For this review, take the finished solid that the model builds, in its own axes (mm). A direction names the side the tool comes from. Round coordinates to 2 decimals unless told otherwise and drop trailing zeros. Order: outer loops, then holes, each group sorted by start corner. A loop starts at its lowest first (then second) coordinate and runs counter-clockwise, first axis right, second up. Notation, with made-up numbers: M -12,75 L 26,75 A24 cw 26,114 Z; hole C 1,19 d7. An arc over 180 degrees is marked long. Answer in a Markdown table with one row per item. Add a question column.
```python
from build123d import *

# Parameters (mm, degrees)
ESQUISSE1_R                         = 20
BOSS_EXTRU_1_DEPTH                  = 430.4
TROU_TARAUD_M81_D                   = 6.8
TROU_TARAUD_M81_DEPTH               = 22.25
TROU_TARAUD_M81_TIP                 = 2.042926105
ENL_V_MAT_EXTRU_1_REACH             = 433.328
ENL_V_MAT_EXTRU_1_DIRECTION_2_DEPTH = 432.328366793
TROU_TARAUD_M41_D                   = 3.3
TROU_TARAUD_M41_DEPTH               = 11.5
TROU_TARAUD_M41_TIP                 = 0.991420021
CHANFREIN1_SIZE                     = 0.8


with BuildPart() as part:
    # Esquisse1 → Boss.-Extru.1 (new body)
    with BuildSketch(Plane(origin=(0, 0, 0), x_dir=(1, 0, 0), z_dir=(0, 1, 0))):
        with Locations(Location((0, 0, 0), (0, 0, 90))):
            Circle(ESQUISSE1_R)
    extrude(amount=BOSS_EXTRU_1_DEPTH)

    # Trou taraudé M81
    with Locations(Plane(origin=(0, 0, 0), x_dir=(-1, 0, 0), z_dir=(0, -1, 0))):
        with Locations((0, -12.5), (0, 12.5)):
            Hole(TROU_TARAUD_M81_D / 2, depth=TROU_TARAUD_M81_DEPTH)
            with Locations((0, 0, -(TROU_TARAUD_M81_DEPTH + TROU_TARAUD_M81_TIP / 2))):  # 118° drill point
                Cone(0, TROU_TARAUD_M81_D / 2, TROU_TARAUD_M81_TIP, mode=Mode.SUBTRACT)

    # Esquisse8 → Enlèv. mat.-Extru.1 (cut, up to next)
    with BuildSketch(Plane.XZ, mode=Mode.PRIVATE) as enl_v_mat_extru_1_sk1:
        with BuildLine():
            Line((-5.5, 19.228884523), (-5.5, 18.9))
            Line((-5.5, 18.9), (5.5, 18.9))
            Line((5.5, 18.9), (5.5, 19.228884523))
            ThreePointArc((5.5, 19.228884523), (0, 20), (-5.5, 19.228884523))
        make_face()
    enl_v_mat_extru_1_tool1 = extrude(enl_v_mat_extru_1_sk1.sketch, amount=-ENL_V_MAT_EXTRU_1_REACH, mode=Mode.PRIVATE) & part.part
    # Esquisse8 → Enlèv. mat.-Extru.1 (cut, up to next)
    with BuildSketch(Plane.XZ, mode=Mode.PRIVATE) as enl_v_mat_extru_1_sk2:
        with BuildLine():
            Line((19.078784028, 6), (15, 6))
            Line((15, 6), (15, -6))
            Line((15, -6), (19.078784028, -6))
            ThreePointArc((19.078784028, -6), (20, 0), (19.078784028, 6))
        make_face()
    enl_v_mat_extru_1_tool2 = extrude(enl_v_mat_extru_1_sk2.sketch, amount=-ENL_V_MAT_EXTRU_1_REACH, mode=Mode.PRIVATE) & part.part
    add(enl_v_mat_extru_1_tool1.solids().sort_by_distance((0, 0, 19.353586))[0], mode=Mode.SUBTRACT)
    add(enl_v_mat_extru_1_tool2.solids().sort_by_distance((17.355884, 0, 0))[0], mode=Mode.SUBTRACT)

    # Esquisse8 → Enlèv. mat.-Extru.1 direction 2 (cut)
    with BuildSketch(Plane.XZ):
        with BuildLine():
            Line((-5.5, 19.228884523), (-5.5, 18.9))
            Line((-5.5, 18.9), (5.5, 18.9))
            Line((5.5, 18.9), (5.5, 19.228884523))
            ThreePointArc((5.5, 19.228884523), (0, 20), (-5.5, 19.228884523))
        make_face()
        with BuildLine():
            Line((19.078784028, 6), (15, 6))
            Line((15, 6), (15, -6))
            Line((15, -6), (19.078784028, -6))
            ThreePointArc((19.078784028, -6), (20, 0), (19.078784028, 6))
        make_face()
    extrude(amount=ENL_V_MAT_EXTRU_1_DIRECTION_2_DEPTH, mode=Mode.SUBTRACT)

    # Trou taraudé M41
    with Locations(Plane(origin=(15, 0, 0), x_dir=(0, 0, -1), z_dir=(1, 0, 0))):
        with Locations((0, 426.4)):
            Hole(TROU_TARAUD_M41_D / 2, depth=TROU_TARAUD_M41_DEPTH)
            with Locations((0, 0, -(TROU_TARAUD_M41_DEPTH + TROU_TARAUD_M41_TIP / 2))):  # 118° drill point
                Cone(0, TROU_TARAUD_M41_D / 2, TROU_TARAUD_M41_TIP, mode=Mode.SUBTRACT)

    # Chanfrein1
    chanfrein1_edges = [part.edges().sort_by_distance(p)[0] for p in [
        (5.5, 430.4, 19.064442262),
        (0, 430.4, 18.9),
        (-5.5, 430.4, 19.064442262),
        (-14.325501649, 430.4, -13.956360647),
        (17.039392014, 430.4, -6),
        (15, 430.4, 0),
        (17.039392014, 430.4, 6),
        (13.956360647, 430.4, 14.325501649),
    ]]
    chamfer(chanfrein1_edges, length=CHANFREIN1_SIZE)


solid = part.part
```
1. The part is to be moulded in two halves that separate along Z. For faces 4 (the conical face through (13.583, 430.272, 13.75)), 5 (the flat face through (-1, 0, 0)), 6 (the cylindrical face through (-0.74, 11.28, 15.82)), say which applies: pulls with the +Z half, pulls with the -Z half, needs draft (parallel to the pull), parting line crosses it, or undercut.
2. For faces 1 (the flat face through (15, 212, 0)), 2 (the cylindrical face through (-0.74, 11.28, -9.18)), 3 (the flat face through (0, 212, 18.9)), list the 3-axis set-ups (+Z, -Z, +X, -X, +Y, -Y) from which the entire face can be reached by the end or side of a thin tool; tool diameter is ignored.
3. To check wall thickness, follow probe 1 along Z at (x, y) = (0, 16); probe 2 along Y at (x, z) = (8.75, 0); probe 3 along X at (y, z) = (13.75, 12.5). State the ranges of each line that lie inside material, in increasing order. Write a range as [from, to].
4. Clearance check with flat-ended pins moving along their axes: pin 1 Ø5 at (y, z) = (310.5, 6.5) entering from +X; pin 2 Ø4.5 at (y, z) = (426.4, 0) entering from +X; pin 3 Ø1.2 at (x, y) = (17.5, 213) entering from +Z; pin 4 Ø4 at (x, z) = (-3.5, 7.5) entering from -Y. State where each tip first meets the part, or that it passes through.
5. Consider section A-A on y = 225.5. Write out the cut boundary in (x, z), plus the area to 3 significant figures.
Solved:
| question | item | result |
|---|---|---|
| 1 | face 4 | pulls with the +Z half |
| 1 | face 5 | needs draft |
| 1 | face 6 | undercut |
| 2 | face 1 | +X, +Y, -Y |
| 2 | face 2 | -Y |
| 2 | face 3 | +Z, +Y, -Y |
| 3 | probe 1 | z = [-20, -15.9], [-9.1, 9.1], [15.9, 18.9] |
| 3 | probe 2 | y = [0, 424.75], [428.05, 430.4] |
| 3 | probe 3 | x = [-15.61, -3.4], [3.4, 15.61] |
| 4 | pin 1 | stops at x = 19.08 |
| 4 | pin 2 | stops at x = 15 |
| 4 | pin 3 | stops at z = 10.7 |
| 4 | pin 4 | stops at y = 0 |
| 5 | outline | M -5.5,18.9 L -5.5,19.23 A20 ccw long 19.08,-6 L 15,-6 L 15,6 L 19.08,6 A20 ccw 5.5,19.23 L 5.5,18.9 Z |
| 5 | area | 1,190 mm^2 |
